Model file for the job. Use its own axes, mm. A direction names the side the tool comes from. Round coordinates to 2 decimals unless told otherwise and drop trailing zeros. Loops run counter-clockwise (first coordinate to the right, second up) from the corner with the lowest first, then second, coordinate; pieces in that order, holes last. Notation, with made-up numbers: (78.25, 79.5) - (113.25, 79.5) arc R16 cw to (113.25, 90.5) - close; hole circle Ø4 at (34.5, -2.5). An arc over 180 degrees is marked (long way). Answer as a JSON object with one key per item and string values.
from build123d import *

# Parameters (mm, degrees)
F1_DEPTH = 9.5
F3_D     = 6.35
F5_D     = 4
F5_DEPTH = 7
F5_TIP   = 1.2017212381
F6_D     = 3.2
F6_DEPTH = 3.5
F6_TIP   = 0.9613769904


with BuildPart() as f1:
    # F0 (on Right) → F1 (new body, symmetric)
    with BuildSketch(Plane.YZ):
        Polygon((-9.2, -4.75), (-9.2, -8.75), (9.2, -8.75), (9.2, -4.75), (4.25, -4.75), (4.25, -0.75), (14.3, -0.75), (14.3, 5.15), (6.75, 5.15), (4.25, 2.65), (-4.25, 2.65), (-6.75, 5.15), (-10.1, 5.15), (-10.1, 6.4), (-8.332233047, 8.167766953), (-9.582233047, 8.167766953), (-13.1, 6.15), (-13.1, 2.15), (-8.65, 2.15), (-4.25, -2.25), (-4.25, -4.75), align=None)
    extrude(amount=F1_DEPTH, both=True)

    # F3 (through all)
    with Locations(Plane(origin=(0, 0, -8.75), x_dir=(1, 0, 0), z_dir=(0, 0, -1))):
        with Locations((0, 0)):
            Hole(F3_D / 2)

    # F5
    with Locations(Plane(origin=(0, 14.3, 0), x_dir=(-1, 0, 0), z_dir=(0, 1, 0))):
        with Locations((0, 2.2)):
            Hole(F5_D / 2, depth=F5_DEPTH)
            with Locations((0, 0, -(F5_DEPTH + F5_TIP / 2))):  # 118° drill point
                Cone(0, F5_D / 2, F5_TIP, mode=Mode.SUBTRACT)

    # F6
    with Locations(Plane(origin=(0, 14.3, 0), x_dir=(-1, 0, 0), z_dir=(0, 1, 0))):
        with Locations((-6, 2.2), (6, 2.2)):
            Hole(F6_D / 2, depth=F6_DEPTH)
            with Locations((0, 0, -(F6_DEPTH + F6_TIP / 2))):  # 118° drill point
                Cone(0, F6_D / 2, F6_TIP, mode=Mode.SUBTRACT)


solid = f1.part
1) Drop flat-ended pins along their axis: P1, Ø2, axis at x = -2.5, y = -11.5, coming from the -Z side; P2, Ø1.7, axis at x = -3.5, y = -8, coming from the +Z side; P3, Ø2, axis at x = -4, z = -3, coming from the +Y side; P4, Ø1.2, axis at x = -4, z = -6.5, coming from the -Y side. Give the stop position or say it passes through.
Values follow:
{"P1": "z = 2.15", "P2": "z = 8.17", "P3": "y = 4.25", "P4": "y = -9.2"}
2) Tool access for faces 1 (the flat face through (0.1, -5.5, 3.9)), 2 (the cylindrical face through (7.48, 12.53, 1.59)), 3 (the flat face through (0, -4.25, -3)): list every direction of +Z, -Z, +X, -X, +Y, -Y with a clear straight run to the whole face (end or side of a thin tool).
Values follow:
{"face 1": "+Z, +X, -X", "face 2": "+Y", "face 3": "+X, -X, -Y"}
3) Slice it at B-B on z = 4.5. List the corners of the cut face in (x, y).
Values follow:
{"outline": "(-9.5, -13.1) - (9.5, -13.1) - (9.5, -6.1) - (-9.5, -6.1) - close; (-9.5, 6.1) - (9.5, 6.1) - (9.5, 14.3) - (-9.5, 14.3) - close"}
4) Slice it at A-A on y = 11.5. List the corners of the cut face in (x, z).
Values follow:
{"outline": "(-9.5, -0.75) - (9.5, -0.75) - (9.5, 5.15) - (-9.5, 5.15) - close; hole circle Ø3.2 at (-6, 2.2); hole circle Ø4 at (0, 2.2); hole circle Ø3.2 at (6, 2.2)"}
5) Two-plate mould, pull along Z, no slides. Class faces 4 (the flat face through (0.13, -11.32, 7.17)), 5 (the flat face through (0.1, -6.5, 0)), 6 (the flat face through (0, 9.2, -7)): pulls with the +Z half, pulls with the -Z half, needs draft (parallel to the pull), parting line crosses it, or undercut.
Values follow:
{"face 4": "pulls with the +Z half", "face 5": "undercut", "face 6": "needs draft"}
6) Slice it at D-D on x = -2.5. List the corners of the cut face in (y, z), then the cut area to 3 significant figures.
Values follow:
{"outline": "(-13.1, 2.15) - (-8.65, 2.15) - (-4.25, -2.25) - (-4.25, -4.75) - (-9.2, -4.75) - (-9.2, -8.75) - (-1.96, -8.75) - (-1.96, 2.65) - (-4.25, 2.65) - (-6.75, 5.15) - (-10.1, 5.15) - (-10.1, 6.4) - (-8.33, 8.17) - (-9.58, 8.17) - (-13.1, 6.15) - close; (1.96, -8.75) - (9.2, -8.75) - (9.2, -4.75) - (4.25, -4.75) - (4.25, -0.75) - (14.3, -0.75) - (14.3, 5.15) - (6.75, 5.15) - (4.25, 2.65) - (1.96, 2.65) - close", "area": "188 mm²"}
7) Probe probe 1 along X at (y, z) = (11.7, 2.2); probe 2 along Z at (x, y) = (0, 10); probe 3 along Z at (x, y) = (-6, 11.65). List the from-to ranges inside material, lowest first.
Values follow:
{"probe 1": "-9.5 to -7.6, -4.4 to -2, 2 to 4.4, 7.6 to 9.5", "probe 2": "-0.75 to 0.2, 4.2 to 5.15", "probe 3": "-0.75 to 0.6, 3.8 to 5.15"}
8) Slice it at C-C on y = -8. List the corners of the cut face in (x, z), then the cut area to 3 significant figures.
Values follow:
{"outline": "(-9.5, -8.75) - (9.5, -8.75) - (9.5, -4.75) - (-9.5, -4.75) - close; (-9.5, 1.5) - (9.5, 1.5) - (9.5, 5.15) - (-9.5, 5.15) - close", "area": "145 mm²"}
